Autodesk Inventor part; units mm, degrees
ref_plane "YZ Plane" through (0, 0, 0) normal (1, 0, 0) x (0, 1, 0)
ref_plane "XZ Plane" through (0, 0, 0) normal (0, 1, 0) x (-1, 0, 0)
ref_plane "XY Plane" through (0, 0, 0) normal (0, 0, 1) x (1, 0, 0)
sketch "Sketch1" plane through (0, 0, 0) normal (0, 1, 0) x (-1, 0, 0)
  line L0 (0, 0) -> (-20, 0)
  line L1 (-20, 0) -> (-20, 10)
  line L2 (-20, 10) -> (0, 10)
  line L3 (0, 10) -> (0, 0)
  dimension "d0" = 20
  dimension "d1" = 10
extrude "Extrusion1" add sketch "Sketch1" along normal blind 5
sketch "Sketch2" plane through (0, 5, 0) normal (0, 1, 0) x (1, 0, 0)
  line L0 (20, 0) -> (0, 0)
  line L1 (4.9996, 0) -> (14.9996, 0)
  line L2 (14.9996, 0) -> (14.9996, -5)
  line L3 (14.9996, -5) -> (4.9996, -5)
  line L4 (4.9996, -5) -> (4.9996, 0)
  dimension "d4" = 10
  dimension "d5" = 5
extrude "Extrusion2" add sketch "Sketch2" along normal blind 8
sketch "Sketch3" plane through (0, 13, 0) normal (0, 1, 0) x (1, 0, 0)
  point P0 (0, 0)
sketch "Sketch4" plane through (4.9996, 5, 5) normal (0, 0, 1) x (1, 0, 0)
  circle A0 centre (5, 5.9999) radius 1
  point P0 (-4.9996, -5)
  dimension "d8" = 2
hole "Hole1" at (9.9996, 10.9999, 5) direction (0, 0, -1) diameter 2 end through all
sketch "Sketch5" plane through (4.9996, 5, 5) normal (0, 0, 1) x (1, 0, 0)
  circle A0 centre (5, 5.9999) radius 1
  line L0 (10, 8) -> (0, 8)
  line L1 (4, 5.9999) -> (5.9994, 5.9999)
  line L2 (5.9994, 5.9999) -> (5.9994, 8)
  line L3 (5.9994, 8) -> (4, 8)
  line L4 (4, 8) -> (4, 5.9999)
  point P0 (-4.9996, -5)
extrude "Extrusion3" cut sketch "Sketch5" against normal blind 5.6375 contours L1 A0 | A0 L4 L0 L2 picked at (5.2495, 6.2209)
sketch "Sketch6" plane through (0, 5, 0) normal (0, 1, 0) x (1, 0, 0)
  circle A0 centre (2.5092, -7.369) radius 0.5
  point P0 (0, 0)
  dimension "d18" = 1
hole "Hole2" at (2.5092, 5, 7.369) direction (0, -1, 0) diameter 1 end through all
sketch "Sketch7" plane through (0, 5, 0) normal (0, 1, 0) x (1, 0, 0)
  circle A0 centre (17.0675, -7.4999) radius 0.5
  point P0 (0, 0)
  dimension "d26" = 1
hole "Hole3" at (17.0675, 5, 7.4999) direction (0, -1, 0) diameter 1 end through all
fillet "Fillet1" radius 0.5 2 edges at (10.999, 13, 2.5) (8.9996, 13, 2.5)
equation "\"d14\" = Thickness"
equation "\"BendRadius\" = Thickness"
equation "\"BendReliefWidth\" = Thickness"
equation "\"BendReliefDepth\" = 0.5 * Thickness"
equation "\"CornerReliefSize\" = 4 * Thickness"
equation "\"MinimumRemnant\" = 2 * Thickness"
equation "\"TransitionRadius\" = BendRadius"
equation "\"JacobiRadiusSize\" = BendRadius"
equation "\"GapSize\" = Thickness"
properties part number "swiatlowod_uchwyt"
Could you check a few things on this model? Use its own coordinates, in mm. A direction names the side the tool comes from. Give positions to 0.01 mm unless a question says otherwise; leave off trailing zeros. Loops run counter-clockwise (first coordinate to the right, second up) from the corner with the lowest first, then second, coordinate; pieces in that order, holes last. Notation, with made-up numbers: (6.25, 38.5) - (14.25, 38.5) arc R16 cw to (14.25, 45.5) - close; hole circle Ø6 at (12, 25). An arc over 180 degrees is marked (long way). Use one line per item in the form item = value.
1. I want a section at A-A (y = 12). Please give me the cut outline in (x, z).
Response values:
outline = (5, 0) - (9, 0) - (9, 5) - (5, 5) - close; (11, 0) - (15, 0) - (15, 5) - (11, 5) - close
2. On a 3-axis mill with a long thin cutter (end or side, diameter ignored), from which of +Z, -Z, +X, -X, +Y, -Y can I reach the whole of each face in a straight line? I mean faces 1 (the face through (10.999, 12, 3)), 2 (the face through (10, 9, 5)), 3 (the face through (10, 5, 0)), 4 (the face through (15, 9, 2)), 5 (the face through (5, 9, 3)). Say none if no direction works.
Response values:
face_1 = +Z, -Z, +Y
face_2 = +Z, +X, -X, +Y
face_3 = -Z, +X, -X, +Y, -Y
face_4 = +Z, -Z, +X, +Y
face_5 = +Z, -Z, -X, +Y
3. I need wall thicknesses on probe 1 along Y at (x, z) = (15.75, 4.75); probe 2 along X at (y, z) = (12.25, 0.5). Which ranges of each line are inside material? Lowest first, please.
Response values:
probe_1 = 0 to 5
probe_2 = 5 to 9, 11 to 15
4. I want a section at D-D (y = 8.75). Please give me the cut outline in (x, z), and give its area (3 significant figures).
Response values:
outline = (5, 0) - (15, 0) - (15, 5) - (5, 5) - close
area = 50.0 mm²
5. I want a section at B-B (z = 2.75). Please give me the cut outline in (x, y), and give its area (3 significant figures).
Response values:
outline = (0, 0) - (20, 0) - (20, 5) - (15, 5) - (15, 13) - (11.5, 13) arc R0.5 ccw to (11, 12.5) - (11, 11) arc R1 cw to (9, 11) - (9, 12.5) arc R0.5 ccw to (8.5, 13) - (5, 13) - (5, 5) - (0, 5) - close
area = 174 mm²
6. I want a section at C-C (x = 8.75). Please give me the cut outline in (y, z), and give its area (3 significant figures).
Response values:
outline = (0, 0) - (12.93, 0) - (12.93, 5) - (5, 5) - (5, 10) - (0, 10) - close
area = 89.7 mm²
7. I'm going to push flat-ended pins straight in: pin 1 Ø1.5 at (y, z) = (9.5, 2.5) entering from -X; pin 2 Ø2.5 at (y, z) = (7.5, 2) entering from +X; pin 3 Ø2.5 at (x, y) = (8.5, 8) entering from +Z. Where does each tip first touch, or does it pass through?
Response values:
pin_1 = 5
pin_2 = 15
pin_3 = 5
